from build123d import *

# Parameters (mm, degrees)
SKETCH2_W           = 51.670795736
SKETCH2_H           = 111.629965862
BOSS_EXTRUDE1_DEPTH = 10
SKETCH3_R           = 4.225
SKETCH3_R_2         = 4.1275
CUT_EXTRUDE1_DEPTH  = 11
SKETCH5_R           = 1.5875
CUT_EXTRUDE2_DEPTH  = 11


with BuildPart() as part:
    # Sketch2 → Boss-Extrude1 (new body)
    with BuildSketch(Plane(origin=(0, 0, 0), x_dir=(0, 0, -1), z_dir=(1, 0, 0))):
        with Locations((416.961058265, -489.879931508)):
            Rectangle(SKETCH2_W, SKETCH2_H)
    extrude(amount=BOSS_EXTRUDE1_DEPTH)

    # Sketch3 → Cut-Extrude1 (cut, through all)
    with BuildSketch(Plane(origin=(10, 0, 0), x_dir=(0, 0, -1), z_dir=(1, 0, 0))):
        with Locations((416.982623845, -460.578730032)):
            Circle(SKETCH3_R)
        with Locations((416.982623845, -519.760730032)):
            Circle(SKETCH3_R)
        with Locations((416.961058265, -489.879931508)):
            Circle(SKETCH3_R_2)
    extrude(amount=-CUT_EXTRUDE1_DEPTH, mode=Mode.SUBTRACT)

    # Sketch5 → Cut-Extrude2 (cut, through all)
    with BuildSketch(Plane(origin=(10, 0, 0), x_dir=(0, 0, -1), z_dir=(1, 0, 0))):
        with Locations((418.78573561, -481.859784241)):
            Circle(SKETCH5_R)
        with Locations((424.981126269, -491.704497776)):
            Circle(SKETCH5_R)
        with Locations((415.136412734, -497.899888435)):
            Circle(SKETCH5_R)
        with Locations((408.941022075, -488.0551749)):
            Circle(SKETCH5_R)
    extrude(amount=-CUT_EXTRUDE2_DEPTH, mode=Mode.SUBTRACT)


solid = part.part
Check sheet for the modelled part. Datum: model origin and axes. Units: mm. Round coordinates to 2 decimals unless told otherwise and drop trailing zeros. Loops run counter-clockwise (first coordinate to the right, second up) from the corner with the lowest first, then second, coordinate; pieces in that order, holes last.
1. Sectioned sample at A-A on x = 7.25. Give the number of separate pieces and of enclosed holes in the cut face, and give its area (3 significant figures).
2. Sectioned sample at B-B on z = -424.5. Record the boundary of the cut face in (x, y), and give its area (3 significant figures).
3. Scan lines: probe 1 along Y at (x, z) = (7, -420); probe 2 along Z at (x, y) = (4.5, -491); probe 3 along Z at (x, y) = (4, -489). Record each from-to range of solid material in increasing order.
4. Mould release check, pull along Z, two halves, no side actions. Record for faces 1 (the flat face through (0, -489, -422)), 2 (the flat face through (5, -491, -442.796)), 3 (the cylindrical face through (5.07, -497.42, -416.65)): released by +Z, released by -Z, zero draft, split by the parting line, or undercut.
Recorded:
1. separate pieces: 1
1. enclosed holes: 7
1. area: 5,570 mm2
2. outline: (0, -545.69) - (10, -545.69) - (10, -493.22) - (0, -493.22) - close; (0, -490.19) - (10, -490.19) - (10, -434.06) - (0, -434.06) - close
2. area: 1,090 mm2
3. probe 1: y = -545.69 to -522.72, -516.8 to -492.67, -487.09 to -482.88, -480.84 to -463.54, -457.62 to -434.06
3. probe 2: z = -442.8 to -426.4, -423.56 to -420.93, -412.99 to -391.13
3. probe 3: z = -442.8 to -420.99, -412.93 to -410.22, -407.67 to -391.13
4. face 1: zero draft
4. face 2: released by -Z
4. face 3: undercut
